```python
from build123d import *

# Parameters (mm, degrees)
SKETCH1_W                      = 76.2
SKETCH1_H                      = 69.85
BOSS_EXTRUDE1_DEPTH            = 31.75
FILLET1_R                      = 9.525
CUT_EXTRUDE1_DEPTH             = 28.575
CUT_EXTRUDE3_DEPTH             = 4.7625
BOSS_EXTRUDE3_DEPTH            = 12.7
F_1_4_CLEARANCE_HOLE2_D        = 6.7564
SKETCH15_W                     = 22.225
SKETCH15_H                     = 19.05
CUT_EXTRUDE5_DEPTH             = 90.634023256
FILLET2_R                      = 5.0165
FILLET3_R                      = 3.429
FILLET4_R                      = 0.508
CHAMFER1_SIZE                  = 3.175
F_2_56_TAPPED_HOLE1_AT_2_COUNT = 2
F_2_56_TAPPED_HOLE1_AT_2_PITCH = 23.188196847
CUT_EXTRUDE4_REACH             = 95.81
SKETCH14_R                     = 6.35
F_4_40_TAPPED_HOLE1_REACH      = 129.201
F_4_40_TAPPED_HOLE1_BORE_R     = 1.1303


with BuildPart() as part:
    # Sketch1 → Boss-Extrude1 (new body)
    with BuildSketch(Plane(origin=(0, 0, 0), x_dir=(1, 0, 0), z_dir=(0, 1, 0))):
        Rectangle(SKETCH1_W, SKETCH1_H)
    extrude(amount=BOSS_EXTRUDE1_DEPTH)

    # Fillet1
    fillet1_edges = [part.edges().sort_by_distance(p)[0] for p in [
        (38.1, 15.875, 34.925),
        (-38.1, 15.875, 34.925),
        (-38.1, 15.875, -34.925),
        (38.1, 15.875, -34.925),
    ]]
    fillet(fillet1_edges, radius=FILLET1_R)

    # Sketch2 → Cut-Extrude1 (cut)
    with BuildSketch(Plane.XZ):
        with BuildLine():
            Line((31.75, -25.4), (31.75, 25.4))
            ThreePointArc((31.75, 25.4), (30.82006403, 27.64506403), (28.575, 28.575))
            Line((28.575, 28.575), (-28.575, 28.575))
            ThreePointArc((-28.575, 28.575), (-30.82006403, 27.64506403), (-31.75, 25.4))
            Line((-31.75, 25.4), (-31.75, -25.4))
            ThreePointArc((-31.75, -25.4), (-30.82006403, -27.64506403), (-28.575, -28.575))
            Line((-28.575, -28.575), (28.575, -28.575))
            ThreePointArc((28.575, -28.575), (30.82006403, -27.64506403), (31.75, -25.4))
        make_face()
    extrude(amount=-CUT_EXTRUDE1_DEPTH, mode=Mode.SUBTRACT)

    # Sketch11 → Cut-Extrude3 (cut)
    with BuildSketch(Plane.XZ):
        with BuildLine():
            Line((36.5125, -25.4), (36.5125, 25.4))
            ThreePointArc((36.5125, 25.4), (34.187660076, 31.012660076), (28.575, 33.3375))
            Line((28.575, 33.3375), (-28.575, 33.3375))
            ThreePointArc((-28.575, 33.3375), (-34.187660076, 31.012660076), (-36.5125, 25.4))
            Line((-36.5125, 25.4), (-36.5125, -25.4))
            ThreePointArc((-36.5125, -25.4), (-34.187660076, -31.012660076), (-28.575, -33.3375))
            Line((-28.575, -33.3375), (28.575, -33.3375))
            ThreePointArc((28.575, -33.3375), (34.187660076, -31.012660076), (36.5125, -25.4))
        make_face()
    extrude(amount=-CUT_EXTRUDE3_DEPTH, mode=Mode.SUBTRACT)

    # Sketch4 → Boss-Extrude3 (add, symmetric)
    with BuildSketch(Plane.XY):
        Polygon((-38.1, 0), (-53.975, 0), (-53.975, 6.35), (-38.1, 25.4), align=None)
    boss_extrude3 = extrude(amount=BOSS_EXTRUDE3_DEPTH, both=True)

    # 1/4 Clearance Hole2 (through all)
    with Locations(Plane(origin=(-13.566959835, 0, 0), x_dir=(1, 0, 0), z_dir=(0, -1, 0))):
        with Locations((-34.058040165, 0)):
            f_1_4_clearance_hole2 = Hole(F_1_4_CLEARANCE_HOLE2_D / 2)

    # Sketch15 → Cut-Extrude5 (cut, through all)
    with BuildSketch(Plane.ZY.offset(38.1)):
        with Locations((0, 15.875)):
            Rectangle(SKETCH15_W, SKETCH15_H)
    cut_extrude5 = extrude(amount=CUT_EXTRUDE5_DEPTH, mode=Mode.SUBTRACT)

    # Mirror4: Boss-Extrude3, 1/4 Clearance Hole2, Cut-Extrude5 across plane
    add(boss_extrude3.mirror(Plane(origin=(0, 0, 0), x_dir=(0, 0, 1), z_dir=(1, 0, 0))))
    add(f_1_4_clearance_hole2.mirror(Plane(origin=(0, 0, 0), x_dir=(0, 0, 1), z_dir=(1, 0, 0))), mode=Mode.SUBTRACT)
    add(cut_extrude5.mirror(Plane(origin=(0, 0, 0), x_dir=(0, 0, 1), z_dir=(1, 0, 0))), mode=Mode.SUBTRACT)

    # Fillet2
    fillet2_edges = [part.edges().sort_by_distance(p)[0] for p in [
        (-38.1, 12.7, -12.7),
        (-38.1, 12.7, 12.7),
        (-38.1, 15.875, 11.1125),
        (-38.1, 15.875, -11.1125),
        (38.1, 12.7, 12.7),
        (38.1, 12.7, -12.7),
        (38.1, 15.875, 11.1125),
        (38.1, 15.875, -11.1125),
    ]]
    fillet(fillet2_edges, radius=FILLET2_R)

    # Fillet3
    fillet3_edges = [part.edges().sort_by_distance(p)[0] for p in [
        (-38.1, 25.4, 11.90625),
        (-38.1, 25.4, -11.90625),
        (38.1, 25.4, -11.90625),
        (38.1, 25.4, 11.90625),
    ]]
    fillet(fillet3_edges, radius=FILLET3_R)

    # Fillet4
    fillet4_edges = [part.edges().sort_by_distance(p)[0] for p in [
        (-53.975, 3.175, -12.7),
        (-53.975, 3.175, 12.7),
        (53.975, 3.175, 12.7),
        (53.975, 3.175, -12.7),
    ]]
    fillet(fillet4_edges, radius=FILLET4_R)

    # Chamfer1
    chamfer1_edges = [part.edges().sort_by_distance(p)[0] for p in [
        (-38.1, 31.75, 0),
        (0, 31.75, -34.925),
        (38.1, 31.75, 0),
        (0, 31.75, 34.925),
        (-35.310192091, 31.75, 32.135192091),
        (35.310192091, 31.75, 32.135192091),
        (35.310192091, 31.75, -32.135192091),
        (-35.310192091, 31.75, -32.135192091),
    ]]
    chamfer(chamfer1_edges, length=CHAMFER1_SIZE)

    # Sketch13 → #2-56 Tapped Hole1 (revolve, cut)
    with BuildSketch(Plane(origin=(-15.875, 4.7625, 30.607), x_dir=(0, 0, -1), z_dir=(1, 0, 0))):
        Polygon((0, 0), (0, 6.12216509), (0.889, 5.588), (0.889, 0), align=None)
    f_2_56_tapped_hole1 = revolve(axis=Axis((-15.875, -1.5875, 30.607), (0, 1, 0)), mode=Mode.SUBTRACT)

    # #2-56 Tapped Hole1 at 2: #2-56 Tapped Hole1 ×2
    with Locations(*[Vector(-0.7722463337018893, 0, -0.6353232248894969) * (i * F_2_56_TAPPED_HOLE1_AT_2_PITCH) for i in range(1, F_2_56_TAPPED_HOLE1_AT_2_COUNT)]):
        add(f_2_56_tapped_hole1, mode=Mode.SUBTRACT)

    # Mirror2: #2-56 Tapped Hole1 across plane
    add(f_2_56_tapped_hole1.mirror(Plane.XY), mode=Mode.SUBTRACT)

    # Mirror2 copy 1 sketch → Mirror2 copy 1 (revolve, cut)
    with BuildSketch(Plane(origin=(-33.782, 4.7625, -15.875), x_dir=(0, 0, 1), z_dir=(1, 0, 0))):
        Polygon((0, 0), (0, -6.12216509), (0.889, -5.588), (0.889, 0), align=None)
    revolve(axis=Axis((-33.782, -1.5875, -15.875), (0, -1, 0)), mode=Mode.SUBTRACT)

    # Mirror3: #2-56 Tapped Hole1 across plane
    add(f_2_56_tapped_hole1.mirror(Plane(origin=(0, 0, 0), x_dir=(0, 0, 1), z_dir=(1, 0, 0))), mode=Mode.SUBTRACT)

    # Mirror3 copy 1 sketch → Mirror3 copy 1 (revolve, cut)
    with BuildSketch(Plane(origin=(33.782, 4.7625, 15.875), x_dir=(0, 0, -1), z_dir=(-1, 0, 0))):
        Polygon((0, 0), (0, -6.12216509), (0.889, -5.588), (0.889, 0), align=None)
    revolve(axis=Axis((33.782, -1.5875, 15.875), (0, -1, 0)), mode=Mode.SUBTRACT)

    # Mirror3 copy 2 sketch → Mirror3 copy 2 (revolve, cut)
    with BuildSketch(Plane(origin=(15.875, 4.7625, -30.607), x_dir=(0, 0, 1), z_dir=(-1, 0, 0))):
        Polygon((0, 0), (0, 6.12216509), (0.889, 5.588), (0.889, 0), align=None)
    revolve(axis=Axis((15.875, -1.5875, -30.607), (0, 1, 0)), mode=Mode.SUBTRACT)

    # Mirror3 copy 3 sketch → Mirror3 copy 3 (revolve, cut)
    with BuildSketch(Plane(origin=(33.782, 4.7625, -15.875), x_dir=(0, 0, 1), z_dir=(-1, 0, 0))):
        Polygon((0, 0), (0, 6.12216509), (0.889, 5.588), (0.889, 0), align=None)
    revolve(axis=Axis((33.782, -1.5875, -15.875), (0, 1, 0)), mode=Mode.SUBTRACT)

    # Sketch14 → Cut-Extrude4 (cut, up to next)
    with BuildSketch(Plane(origin=(0, 0, -34.925), x_dir=(-1, 0, 0), z_dir=(0, 0, -1)), mode=Mode.PRIVATE) as cut_extrude4_sk1:
        with Locations((-15.875, 15.875)):
            Circle(SKETCH14_R)
    cut_extrude4_tool1 = extrude(cut_extrude4_sk1.sketch, amount=-CUT_EXTRUDE4_REACH, mode=Mode.PRIVATE) & part.part
    # Sketch14 → Cut-Extrude4 (cut, up to next)
    with BuildSketch(Plane(origin=(0, 0, -34.925), x_dir=(-1, 0, 0), z_dir=(0, 0, -1)), mode=Mode.PRIVATE) as cut_extrude4_sk2:
        with Locations((15.875, 15.875)):
            Circle(SKETCH14_R)
    cut_extrude4_tool2 = extrude(cut_extrude4_sk2.sketch, amount=-CUT_EXTRUDE4_REACH, mode=Mode.PRIVATE) & part.part
    add(cut_extrude4_tool1.solids().sort_by_distance((15.875, 15.875, -34.925))[0], mode=Mode.SUBTRACT)
    add(cut_extrude4_tool2.solids().sort_by_distance((-15.875, 15.875, -34.925))[0], mode=Mode.SUBTRACT)

    # #4-40 Tapped Hole1 bore → #4-40 Tapped Hole1 (cut, up to next)
    with BuildSketch(Plane(origin=(-13.435602358, -50.449576404, -34.925), x_dir=(-1, 0, 0), z_dir=(0, 0, -1)), mode=Mode.PRIVATE) as f_4_40_tapped_hole1_sk1:
        with Locations((-5.104402358, 73.868376404)):
            Circle(F_4_40_TAPPED_HOLE1_BORE_R)
    f_4_40_tapped_hole1_tool1 = extrude(f_4_40_tapped_hole1_sk1.sketch, amount=-F_4_40_TAPPED_HOLE1_REACH, mode=Mode.PRIVATE) & part.part
    # #4-40 Tapped Hole1 bore → #4-40 Tapped Hole1 (cut, up to next)
    with BuildSketch(Plane(origin=(-13.435602358, -50.449576404, -34.925), x_dir=(-1, 0, 0), z_dir=(0, 0, -1)), mode=Mode.PRIVATE) as f_4_40_tapped_hole1_sk2:
        with Locations((9.983197642, 73.868376404)):
            Circle(F_4_40_TAPPED_HOLE1_BORE_R)
    f_4_40_tapped_hole1_tool2 = extrude(f_4_40_tapped_hole1_sk2.sketch, amount=-F_4_40_TAPPED_HOLE1_REACH, mode=Mode.PRIVATE) & part.part
    # #4-40 Tapped Hole1 bore → #4-40 Tapped Hole1 (cut, up to next)
    with BuildSketch(Plane(origin=(-13.435602358, -50.449576404, -34.925), x_dir=(-1, 0, 0), z_dir=(0, 0, -1)), mode=Mode.PRIVATE) as f_4_40_tapped_hole1_sk3:
        with Locations((9.983197642, 58.780776404)):
            Circle(F_4_40_TAPPED_HOLE1_BORE_R)
    f_4_40_tapped_hole1_tool3 = extrude(f_4_40_tapped_hole1_sk3.sketch, amount=-F_4_40_TAPPED_HOLE1_REACH, mode=Mode.PRIVATE) & part.part
    # #4-40 Tapped Hole1 bore → #4-40 Tapped Hole1 (cut, up to next)
    with BuildSketch(Plane(origin=(-13.435602358, -50.449576404, -34.925), x_dir=(-1, 0, 0), z_dir=(0, 0, -1)), mode=Mode.PRIVATE) as f_4_40_tapped_hole1_sk4:
        with Locations((-5.104402358, 58.780776404)):
            Circle(F_4_40_TAPPED_HOLE1_BORE_R)
    f_4_40_tapped_hole1_tool4 = extrude(f_4_40_tapped_hole1_sk4.sketch, amount=-F_4_40_TAPPED_HOLE1_REACH, mode=Mode.PRIVATE) & part.part
    # #4-40 Tapped Hole1 bore → #4-40 Tapped Hole1 (cut, up to next)
    with BuildSketch(Plane(origin=(-13.435602358, -50.449576404, -34.925), x_dir=(-1, 0, 0), z_dir=(0, 0, -1)), mode=Mode.PRIVATE) as f_4_40_tapped_hole1_sk5:
        with Locations((-21.766802358, 58.780776404)):
            Circle(F_4_40_TAPPED_HOLE1_BORE_R)
    f_4_40_tapped_hole1_tool5 = extrude(f_4_40_tapped_hole1_sk5.sketch, amount=-F_4_40_TAPPED_HOLE1_REACH, mode=Mode.PRIVATE) & part.part
    # #4-40 Tapped Hole1 bore → #4-40 Tapped Hole1 (cut, up to next)
    with BuildSketch(Plane(origin=(-13.435602358, -50.449576404, -34.925), x_dir=(-1, 0, 0), z_dir=(0, 0, -1)), mode=Mode.PRIVATE) as f_4_40_tapped_hole1_sk6:
        with Locations((-21.766802358, 73.868376404)):
            Circle(F_4_40_TAPPED_HOLE1_BORE_R)
    f_4_40_tapped_hole1_tool6 = extrude(f_4_40_tapped_hole1_sk6.sketch, amount=-F_4_40_TAPPED_HOLE1_REACH, mode=Mode.PRIVATE) & part.part
    # #4-40 Tapped Hole1 bore → #4-40 Tapped Hole1 (cut, up to next)
    with BuildSketch(Plane(origin=(-13.435602358, -50.449576404, -34.925), x_dir=(-1, 0, 0), z_dir=(0, 0, -1)), mode=Mode.PRIVATE) as f_4_40_tapped_hole1_sk7:
        with Locations((-36.854402358, 73.868376404)):
            Circle(F_4_40_TAPPED_HOLE1_BORE_R)
    f_4_40_tapped_hole1_tool7 = extrude(f_4_40_tapped_hole1_sk7.sketch, amount=-F_4_40_TAPPED_HOLE1_REACH, mode=Mode.PRIVATE) & part.part
    # #4-40 Tapped Hole1 bore → #4-40 Tapped Hole1 (cut, up to next)
    with BuildSketch(Plane(origin=(-13.435602358, -50.449576404, -34.925), x_dir=(-1, 0, 0), z_dir=(0, 0, -1)), mode=Mode.PRIVATE) as f_4_40_tapped_hole1_sk8:
        with Locations((-36.854402358, 58.780776404)):
            Circle(F_4_40_TAPPED_HOLE1_BORE_R)
    f_4_40_tapped_hole1_tool8 = extrude(f_4_40_tapped_hole1_sk8.sketch, amount=-F_4_40_TAPPED_HOLE1_REACH, mode=Mode.PRIVATE) & part.part
    add(f_4_40_tapped_hole1_tool1.solids().sort_by_distance((-8.3312, 23.4188, -34.925))[0], mode=Mode.SUBTRACT)
    add(f_4_40_tapped_hole1_tool2.solids().sort_by_distance((-23.4188, 23.4188, -34.925))[0], mode=Mode.SUBTRACT)
    add(f_4_40_tapped_hole1_tool3.solids().sort_by_distance((-23.4188, 8.3312, -34.925))[0], mode=Mode.SUBTRACT)
    add(f_4_40_tapped_hole1_tool4.solids().sort_by_distance((-8.3312, 8.3312, -34.925))[0], mode=Mode.SUBTRACT)
    add(f_4_40_tapped_hole1_tool5.solids().sort_by_distance((8.3312, 8.3312, -34.925))[0], mode=Mode.SUBTRACT)
    add(f_4_40_tapped_hole1_tool6.solids().sort_by_distance((8.3312, 23.4188, -34.925))[0], mode=Mode.SUBTRACT)
    add(f_4_40_tapped_hole1_tool7.solids().sort_by_distance((23.4188, 23.4188, -34.925))[0], mode=Mode.SUBTRACT)
    add(f_4_40_tapped_hole1_tool8.solids().sort_by_distance((23.4188, 8.3312, -34.925))[0], mode=Mode.SUBTRACT)


solid = part.part
```
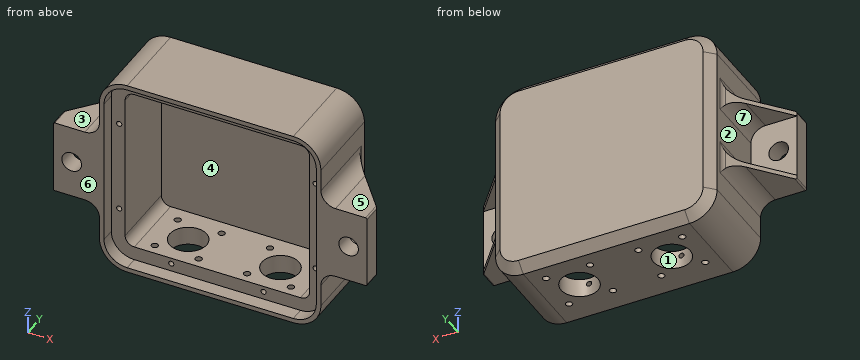
Source: CAD feature listing. Evaluate the final solid. Frame: model axes, mm. Face numbers are marked on the shaded views. A direction names the side the tool comes from. Give positions to 0.01 mm unless a question says otherwise; leave off trailing zeros.
(1) Material intervals for line 1 along X through (y, z) = (18, 18); line 2 along Z through (x, y) = (18, 7) (3 decimals); line 3 along X through (y, z) = (18, -30.5), sorted ascending.
(2) Access query for the marked faces 1, 2, 3 and 4. Directions: +Z, -Z, +X, -X, +Y, -Y. A direction counts if a zero-diameter tool reaches every point of the face in a straight line with its end or side. Return the directions, or none.
(3) Pull-direction query (Z, two-part tool) for the marked faces 5, 6 and 7; classes: +Z half, -Z half, draft (parallel to the pull), parting line (faces both ways), or undercut.
(4) Section query A-A (z = 0). State how many separate pieces and enclosed holes the cut face has, plus the area to 3 significant figures.
(5) Contact query for flat-ended pins moving along their axis: P1, Ø6, axis at y = 25.5, z = 16, coming from the -X side; P2, Ø10, axis at y = 24, z = -10, coming from the +X side; P3, Ø11, axis at x = 47.625, z = 0, coming from the +Y side. Output: stop coordinate, or through.
Outcome:
1. line 1: x = -38.1 to -31.75, 31.75 to 38.1
1. line 2: z = -34.925 to -28.575, 28.575 to 34.925
1. line 3: x = -36.62 to -21.86, -9.89 to 9.89, 21.86 to 36.62
2. face 1: -Z
2. face 2: -X, +Y
2. face 3: +Z, -X, +Y, -Y
2. face 4: -Y
3. face 5: +Z half
3. face 6: draft
3. face 7: undercut
4. separate pieces: 3
4. enclosed holes: 0
4. area: 665 mm2
5. P1: stops at x = -39.83
5. P2: stops at x = 43.33
5. P3: stops at y = 6.35
